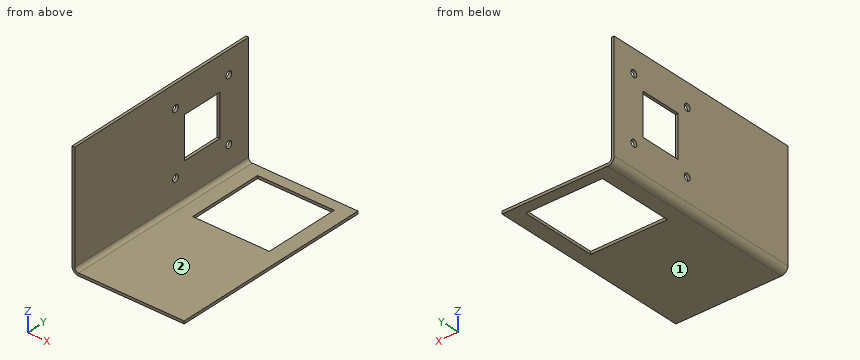
Autodesk Inventor part; units mm, degrees
ref_plane "YZ Plane" through (0, 0, 0) normal (1, 0, 0) x (0, 1, 0)
ref_plane "XZ Plane" through (0, 0, 0) normal (0, 1, 0) x (-1, 0, 0)
ref_plane "XY Plane" through (0, 0, 0) normal (0, 0, 1) x (1, 0, 0)
sketch "Sketch1" plane through (0, 0, 0) normal (0, 0, 1) x (1, 0, 0)
  line L0 (-41, -75) -> (41, -75)
  line L1 (41, -75) -> (41, 75)
  line L2 (41, 75) -> (-41, 75)
  line L3 (-41, 75) -> (-41, -75)
  line L4 (-41, -75) -> (41, 75) construction
  line L5 (41, -75) -> (-41, 75) construction
  point P0 (0, 0)
  dimension "d154" = 82
  dimension "d155" = 150
extrude "Plate5" add sketch "Sketch1" along normal blind 2
sketch "Sketch7" plane through (-39, -75, 0) normal (-1, 0, 0) x (0, -1, 0)
  line L0 (-150, 0) -> (0, 0)
  line L1 (0, 0) -> (0, 84)
  line L2 (0, 84) -> (-150, 84)
  line L3 (-150, 84) -> (-150, 0)
edge flange "Flange3" height 84 angle 90 thickness 2 bend radius 2.75 thickness toward (-1, 0, 0) relief round relief width 2 relief depth 1 edges at (-41, 0, 2) wall of the first edge with corners at (-39, 75, 0) (-39, -75, 0) (-39, -75, 84) (-39, 75, 84)
bend "Bend3"
corner "Corner3"
sketch "Sketch8" plane through (0, 0, 2) normal (0, 0, 1) x (1, 0, 0)
  line L0 (41, 75) -> (41, -75)
  line L1 (-36.25, 75) -> (41, 75)
  line L2 (30.375, 67) -> (-25.625, 67)
  line L3 (-25.625, 67) -> (-25.625, 11)
  line L4 (-25.625, 11) -> (30.375, 11)
  line L5 (30.375, 11) -> (30.375, 67)
  line L6 (30.375, 67) -> (-25.625, 11) construction
  line L7 (-25.625, 67) -> (30.375, 11) construction
  point P0 (0, 0)
  point P1 (2.375, 39)
  point P2 (2.375, 75)
  dimension "d167" = 56
  dimension "d168" = 56
  dimension "d169" = 8
extrude "Cut1" cut sketch "Sketch8" against normal blind 2
sketch "Sketch9" plane through (-41, -75, 84) normal (-1, 0, 0) x (0, 0, 1)
  line L0 (-24.375, 94.75) -> (-54.875, 94.75)
  line L1 (-54.875, 94.75) -> (-54.875, 125.25)
  line L2 (-54.875, 125.25) -> (-24.375, 125.25)
  line L3 (-24.375, 125.25) -> (-24.375, 94.75)
  line L4 (-24.375, 94.75) -> (-54.875, 125.25) construction
  line L5 (-54.875, 94.75) -> (-24.375, 125.25) construction
  circle A0 centre (-16.625, 87) radius 2.5
  circle A1 centre (-62.625, 87) radius 2.5
  circle A2 centre (-62.625, 133) radius 2.5
  circle A3 centre (-16.625, 133) radius 2.5
  circle A4 centre (-39.625, 110) radius 32.5269 construction
  line L6 (-54.875, 94.75) -> (-62.625, 87) construction
  line L7 (-14.125, 84.5) -> (-65.125, 84.5) construction
  line L8 (-65.125, 84.5) -> (-65.125, 135.5) construction
  line L9 (-65.125, 135.5) -> (-14.125, 135.5) construction
  line L10 (-14.125, 135.5) -> (-14.125, 84.5) construction
  line L11 (-14.125, 84.5) -> (-65.125, 135.5) construction
  line L12 (-65.125, 84.5) -> (-14.125, 135.5) construction
  line L13 (-79.25, 150) -> (0, 150)
  line L14 (-39.625, 150) -> (-39.625, 110) construction
  circle A5 centre (-62.625, 133) radius 10.9602 construction
  line L15 (-16.625, 87) -> (-62.625, 87) construction
  line L16 (-62.625, 87) -> (-62.625, 133) construction
  line L17 (-62.625, 133) -> (-16.625, 133) construction
  line L18 (-16.625, 133) -> (-16.625, 87) construction
  line L19 (-16.625, 87) -> (-62.625, 133) construction
  line L20 (-62.625, 87) -> (-16.625, 133) construction
  point P0 (-84, 75)
  point P1 (-104.8197, 150.8767)
  point P2 (-104.8197, 150.8767)
  dimension "d181" = 21.9203
  dimension "d174" = 30.5
  dimension "d175" = 30.5
  dimension "d176" = 5
  dimension "d179" = 40
  dimension "d180" = 51
  dimension "d184" = 46
extrude "Cut2" cut sketch "Sketch9" against normal blind 2
properties part number "SLM 1652 FDS Central tube wall" material "Stainless Steel"
Here's how the part is built. I have some questions about the finished solid (model axes, mm). Face numbers are marked on the shaded views. A direction names the side the tool comes from. Coordinates: 2 decimals unless noted, no trailing zeros. Loops run counter-clockwise (first coordinate to the right, second up) from the corner with the lowest first, then second, coordinate; pieces in that order, holes last. Notation, with made-up numbers: (28, 0.25) - (32, 0.25) arc R27 cw to (32, 18.25) - close; hole circle Ø3 at (64.5, -20.5). An arc over 180 degrees is marked (long way). Return JSON: item names as keys, results as strings. Group by question number.
Item 1: Will these pins go through, and if not, where does the flat tip stop? P1, Ø1, axis at y = -0.5, z = 34.5, coming from the +X side; P2, Ø6, axis at y = 12, z = 21.375, coming from the -X side; P3, Ø6, axis at x = -30, y = -4.5, coming from the +Z side; P4, Ø1, axis at y = 29.5, z = 1, coming from the -X side.
Item 2: If we section it at C-C on y = 58: Write out the boundary of the cut face in (x, z) (3 decimals), and give its area (3 significant figures).
Item 3: I need wall thicknesses on line 1 (Z direction, x = -26, y = -10.5); line 2 (X direction, y = -22, z = 76.5). Which ranges of each line are inside material? Lowest first, please. Write a range as from..to.
Item 4: If we section it at D-D on y = -46.5: Write out the boundary of the cut face in (x, z).
Item 5: On a 3-axis mill with a long thin cutter (end or side, diameter ignored), from which of +Z, -Z, +X, -X, +Y, -Y can I reach the whole of each face in a straight line? I mean the marked faces 1 and 2. Say none if no direction works.
Item 6: If we section it at B-B on z = 32: Write out the boundary of the cut face in (x, y), and give its area (3 significant figures).
Item 7: If we section it at A-A on x = -10.5: Write out the boundary of the cut face in (y, z), and give its area (3 significant figures).
Calculated:
{
 "1": {"P1": "stops at x = -39", "P2": "stops at x = -41", "P3": "stops at z = 2", "P4": "stops at x = -39.71"},
 "2": {"outline": "(-41, 4.75) arc R4.75 ccw to (-36.25, 0) - (-25.625, 0) - (-25.625, 2) - (-36.25, 2) arc R2.75 cw to (-39, 4.75) - (-39, 18.875) - (-41, 18.875) - close; (-41, 23.875) - (-39, 23.875) - (-39, 64.875) - (-41, 64.875) - close; (-41, 69.875) - (-39, 69.875) - (-39, 84) - (-41, 84) - close; (30.375, 0) - (41, 0) - (41, 2) - (30.375, 2) - close", "area": "193 mm^2"},
 "3": {"line 1": "z = 0..2", "line 2": "x = -41..-39"},
 "4": {"outline": "(-41, 4.75) arc R4.75 ccw to (-36.25, 0) - (41, 0) - (41, 2) - (-36.25, 2) arc R2.75 cw to (-39, 4.75) - (-39, 84) - (-41, 84) - close"},
 "5": {"face 1": "-Z, +X, -X, +Y, -Y", "face 2": "+Z, +X, +Y, -Y"},
 "6": {"outline": "(-41, -75) - (-39, -75) - (-39, 19.75) - (-41, 19.75) - close; (-41, 50.25) - (-39, 50.25) - (-39, 75) - (-41, 75) - close", "area": "239 mm^2"},
 "7": {"outline": "(-75, 0) - (11, 0) - (11, 2) - (-75, 2) - close; (67, 0) - (75, 0) - (75, 2) - (67, 2) - close", "area": "188 mm^2"}
}
